```python
from build123d import *

# Parameters (mm, degrees)
SKETCH1_W           = 50
SKETCH1_H           = 54.105
BOSS_EXTRUDE1_DEPTH = 12
SKETCH2_R           = 3.15
CUT_EXTRUDE1_DEPTH  = 75.641483272
FILLET1_R           = 8
SKETCH3_R           = 12
SKETCH3_R_2         = 1.7
CUT_EXTRUDE2_DEPTH  = 75.641483272
CUT_EXTRUDE4_DEPTH  = 8
CHAMFER1_SIZE       = 0.5


with BuildPart() as part:
    # Sketch1 → Boss-Extrude1 (new body)
    with BuildSketch(Plane.XY):
        with Locations((25, 27.0525)):
            Rectangle(SKETCH1_W, SKETCH1_H)
    extrude(amount=BOSS_EXTRUDE1_DEPTH)

    # Sketch2 → Cut-Extrude1 (cut, through all)
    with BuildSketch(Plane(origin=(0, 0, 0), x_dir=(0, 0, -1), z_dir=(1, 0, 0))):
        with Locations((-6, 46.105)):
            Circle(SKETCH2_R)
        with Locations(Location((-6, 8, 0), (0, 0, 180))):
            Circle(SKETCH2_R)
    extrude(amount=CUT_EXTRUDE1_DEPTH, mode=Mode.SUBTRACT)

    # Fillet1
    fillet1_edges = [part.edges().sort_by_distance(p)[0] for p in [
        (25, 54.105, 0),
        (25, 0, 0),
    ]]
    fillet(fillet1_edges, radius=FILLET1_R)

    # Sketch3 → Cut-Extrude2 (cut, through all)
    with BuildSketch(Plane(origin=(0, 0, 0), x_dir=(-1, 0, 0), z_dir=(0, 0, -1))):
        with Locations((-32, 27.0525)):
            Circle(SKETCH3_R)
        with Locations((-19, 40.0525)):
            Circle(SKETCH3_R_2)
        with Locations((-19, 14.0525)):
            Circle(SKETCH3_R_2)
        with Locations((-45, 14.0525)):
            Circle(SKETCH3_R_2)
        with Locations((-45, 40.0525)):
            Circle(SKETCH3_R_2)
        with BuildLine():
            Line((-8.5, 0), (-8.5, 24.282572203))
            ThreePointArc((-8.5, 24.282572203), (-10.15, 27.0525), (-8.5, 29.822427797))
            Line((-8.5, 29.822427797), (-8.5, 33.0525))
            ThreePointArc((-8.5, 33.0525), (-7, 34.5525), (-5.5, 33.0525))
            Line((-5.5, 33.0525), (-5.5, 29.822427797))
            ThreePointArc((-5.5, 29.822427797), (-3.85, 27.0525), (-5.5, 24.282572203))
            Line((-5.5, 24.282572203), (-5.5, 0))
            Line((-5.5, 0), (-8.5, 0))
        make_face()
    extrude(amount=-CUT_EXTRUDE2_DEPTH, mode=Mode.SUBTRACT)

    # Sketch5 → Cut-Extrude4 (cut)
    with BuildSketch(Plane(origin=(0, 0, 0), x_dir=(-1, 0, 0), z_dir=(0, 0, -1))):
        with BuildLine():
            Line((-19, 17.6525), (-14, 17.6525))
            Line((-14, 17.6525), (-14, 36.4525))
            Line((-14, 36.4525), (-19, 36.4525))
            ThreePointArc((-19, 36.4525), (-21.510876341, 37.472674425), (-22.598679445, 39.955))
            Line((-22.598679445, 39.955), (-22.598679445, 41.7525))
            Line((-22.598679445, 41.7525), (-41.401320555, 41.7525))
            Line((-41.401320555, 41.7525), (-41.401320555, 39.955))
            ThreePointArc((-41.401320555, 39.955), (-42.489123659, 37.472674425), (-45, 36.4525))
            Line((-45, 36.4525), (-50, 36.4525))
            Line((-50, 36.4525), (-50, 17.6525))
            Line((-50, 17.6525), (-45, 17.6525))
            ThreePointArc((-45, 17.6525), (-42.489123659, 16.632325575), (-41.401320555, 14.15))
            Line((-41.401320555, 14.15), (-41.401320555, 12.3525))
            Line((-41.401320555, 12.3525), (-22.598679445, 12.3525))
            Line((-22.598679445, 12.3525), (-22.598679445, 14.15))
            ThreePointArc((-22.598679445, 14.15), (-21.510876341, 16.632325575), (-19, 17.6525))
        make_face()
    extrude(amount=-CUT_EXTRUDE4_DEPTH, mode=Mode.SUBTRACT)

    # Chamfer1
    chamfer1_edges = [part.edges().sort_by_distance(p)[0] for p in [
        (50, 27.0525, 12),
        (25, 54.105, 12),
        (0, 27.0525, 12),
        (29.25, 0, 12),
        (10.15, 27.0525, 12),
        (8.5, 31.437463898, 12),
        (7, 34.5525, 12),
        (5.5, 31.437463898, 12),
        (3.85, 27.0525, 12),
        (5.5, 12.141286102, 12),
        (8.5, 12.141286102, 12),
        (44, 27.0525, 12),
        (2.75, 0, 12),
        (20.7, 14.0525, 12),
        (46.7, 40.0525, 12),
    ]]
    chamfer(chamfer1_edges, length=CHAMFER1_SIZE)


solid = part.part
```
Here's how the part is built. I have some questions about the finished solid (model axes, mm). A direction names the side the tool comes from. Coordinates: 2 decimals unless noted, no trailing zeros.
1) Imagine slicing it at A-A on x = 32. State how many separate pieces and enclosed holes the cut face has, and give its area (3 significant figures).
2) Will these pins go through, and if not, where does the flat tip stop? pin 1 (1 mm diameter, centred on x = 36.5, y = 12.5, fed in from -Z); pin 2 (1.5 mm diameter, centred on x = 16, z = 4.5, fed in from +Y); pin 3 (9 mm diameter, centred on x = 36.5, y = 20, fed in from -Z); pin 4 (1.5 mm diameter, centred on x = 48.5, z = 5, fed in from +Y).
3) We'd pull the mould along Y, two halves only. Please class faces 1 (the face through (25.35, 51.7, 2.28)), 2 (the face through (14, 27, 4)), 3 (the face through (3.85, 27.1, 5.67)), 4 (the face through (50, 26.7, 8.2)): +Y half, -Y half, draft (parallel to the pull), parting line (faces both ways), or undercut.
4) Which directions (+Z, -Z, +X, -X, +Y, -Y) give clear straight access to the entire face, cutting with the end or side of a thin tool? Please do faces 5 (the face through (42.52, 16.66, 3.94)), 6 (the face through (26.46, 16.41, 9.73)), 7 (the face through (47, 36.452, 4)).
5) I need wall thicknesses on line 1 (Y direction, x = 40, z = 4.5); line 2 (Y direction, x = 16.5, z = 5.75); line 3 (Y direction, x = 2.5, z = 6) (3 decimals). Which ranges of each line are inside material? Lowest first, please.
Response values:
1. separate pieces: 2
1. enclosed holes: 2
1. area: 228 mm2
2. pin 1: stops at z = 0
2. pin 2: stops at y = 53.62
2. pin 3: stops at z = 8
2. pin 4: stops at y = 53.78
3. face 1: +Y half
3. face 2: undercut
3. face 3: undercut
3. face 4: draft
4. face 5: -Z
4. face 6: +Z, -Z
4. face 7: -Z, +X
5. line 1: y = 0.81 to 5.23, 10.77 to 12.35, 41.75 to 43.34, 48.87 to 53.3
5. line 2: y = 0.32 to 4.86, 11.14 to 17.65, 36.45 to 42.96, 49.25 to 53.78
5. line 3: y = 0.254 to 4.85, 11.15 to 42.955, 49.255 to 53.851
